Build history of the part. All positions in model axes, mm. A direction names the side the tool comes from. Round coordinates to 2 decimals unless told otherwise and drop trailing zeros. Order: outer loops, then holes, each group sorted by start corner. A loop starts at its lowest first (then second) coordinate and runs counter-clockwise, first axis right, second up. Notation, with made-up numbers: (75.25, 46) -> (84.25, 46) arc R20 cw to (84.25, 82) -> close; hole circle Ø4 at (-3, -3.75). An arc over 180 degrees is marked (long way). Use a Markdown table: item, result. Add a question column.
Item 1: Two-plate mould, pull along X, no slides. Class faces 1 (the face through (9.45, -10, 6)), 2 (the face through (0, 0, -1)), 3 (the face through (0, -15, 16.939)): released by +X, released by -X, zero draft, split by the parting line, or undercut.
Item 2: Slice it at D-D, the plane y = 9.5. Give the cut face in (x, z).
Item 3: Slice it at B-B, the plane z = 10. Give the cut face in (x, y), plus the area to 3 significant figures.
Item 4: Probe L1, parallel to X at y = 7.75, z = 0; L2, parallel to X at y = -13, z = -0.5; L3, parallel to Y at x = 8, z = 5. List the from-to ranges inside material, lowest first.
Item 5: 3-axis set-ups, long thin cutter, end or side, ignore diameter. For faces 4 (the face through (-8.75, 7, -13)), 5 (the face through (-0.141, -7.782, 16.573)), 6 (the face through (0, -10, -1.961)), 7 (the face through (-9.45, -10, 5)): which of +Z, -Z, +X, -X, +Y, -Y reach the whole face in a straight line?
Item 6: Pin check, flat tips, straight feed: pin 1 (12 mm diameter, centred on y = -12.5, z = 3.5, fed in from +X); pin 2 (2.5 mm diameter, centred on y = 3.5, z = -13, fed in from -X); pin 3 (2 mm diameter, centred on x = -9, y = 2.5, fed in from +Z). Stop position of each tip, or through.
Item 7: Slice it at A-A, the plane y = -14. Give the cut face in (x, z), plus the area to 3 significant figures.
Autodesk Inventor part; units mm, degrees
ref_plane "YZ Plane" through (0, 0, 0) normal (1, 0, 0) x (0, 1, 0)
ref_plane "XZ Plane" through (0, 0, 0) normal (0, 1, 0) x (-1, 0, 0)
ref_plane "XY Plane" through (0, 0, 0) normal (0, 0, 1) x (1, 0, 0)
sketch "Sketch1" plane through (0, 0, 0) normal (0, 1, 0) x (-1, 0, 0)
  circle A0 centre (0, 0) radius 14.15
  circle A1 centre (0, 0) radius 16.574
  dimension "d0" = 28.3
  dimension "d1" = 2.424
extrude "Extrusion1" add sketch "Sketch1" along normal blind 13
sketch "Sketch2" plane through (0, 0, 0) normal (0, -1, 0) x (1, 0, 0)
  circle A0 centre (0, 0) radius 16.574
extrude "Extrusion2" add sketch "Sketch2" along normal blind 3
sketch "Sketch3" plane through (0, 13, 0) normal (0, 1, 0) x (1, 0, 0)
  line L0 (0, 16.574) -> (-8.75, 16.574)
  line L1 (-8.75, 16.574) -> (8.75, 16.574)
  line L2 (-8.75, 16.574) -> (8.75, 16.574)
  line L3 (8.75, 16.574) -> (8.75, 5.314)
  line L4 (8.75, 5.314) -> (-8.75, 5.314)
  line L5 (-8.75, 5.314) -> (-8.75, 16.574)
  dimension "d6" = 8.75
  dimension "d7" = 17.5
extrude "Extrusion3" cut sketch "Sketch3" against normal up to surface (13 mm away)
sketch "Sketch4" plane through (0, -3, 0) normal (0, -1, 0) x (1, 0, 0)
  arc A0 (8.75, -14.076) -> (-8.75, -14.076) centre (0, 0) ccw
  line L0 (0, 16.574) -> (0, 2.9438)
  line L1 (0, 2.9438) -> (0, 12.0338)
  line L2 (-9.45, -1.9612) -> (-9.45, 16.9388)
  line L3 (-9.45, 16.9388) -> (9.45, 16.9388)
  line L4 (9.45, 16.9388) -> (9.45, -1.9612)
  line L5 (9.45, -1.9612) -> (-9.45, -1.9612)
  point P0 (0.0791, 7.4888)
  point P1 (0, 7.4888)
  point P2 (0, -1.9612)
  dimension "d13" = 18.9
extrude "Extrusion4" add sketch "Sketch4" along normal blind 14.7
sketch "Sketch5" plane through (0, -3, 0) normal (0, 1, 0) x (1, 0, 0)
  arc A0 (-9.45, -13.616) -> (9.45, -13.616) centre (0, 0) ccw
  line L0 (-9.45, -13.616) -> (-9.45, -16.9388)
  line L1 (-9.45, -16.9388) -> (9.45, -16.9388)
  line L2 (9.45, -16.9388) -> (9.45, -13.616)
extrude "Extrusion5" cut sketch "Sketch5" against normal blind 9.7
properties part number "stepper_housing"
Check sheet entries:
| question | item | result |
|---|---|---|
| 1 | face 1 | released by +X |
| 1 | face 2 | undercut |
| 1 | face 3 | zero draft |
| 2 | outline | (-8.75, -14.08) -> (-8.75, -11.12) arc R14.15 cw (long way) to (8.75, -11.12) -> (8.75, -14.08) arc R16.57 ccw (long way) to start |
| 3 | outline | (-13.22, -3) -> (-9.45, -3) -> (-9.45, -17.7) -> (9.45, -17.7) -> (9.45, -3) -> (13.22, -3) -> (13.22, 13) -> (10.01, 13) -> (10.01, 0) -> (-10.01, 0) -> (-10.01, 13) -> (-13.22, 13) -> close |
| 3 | area | 440 mm2 |
| 4 | L1 | -16.57 to -14.15, 14.15 to 16.57 |
| 4 | L2 | -9.45 to 9.45 |
| 4 | L3 | -17.7 to 0 |
| 5 | face 4 | -Z, +Y |
| 5 | face 5 | +Z, +Y |
| 5 | face 6 | -Z, +X, -X, -Y |
| 5 | face 7 | +Z, -Z, -X, -Y |
| 6 | pin 1 | x = 9.45 |
| 6 | pin 2 | x = -11.69 |
| 6 | pin 3 | z = 14.52 |
| 7 | outline | (-9.45, -1.96) -> (9.45, -1.96) -> (9.45, 16.94) -> (-9.45, 16.94) -> close |
| 7 | area | 357 mm2 |
